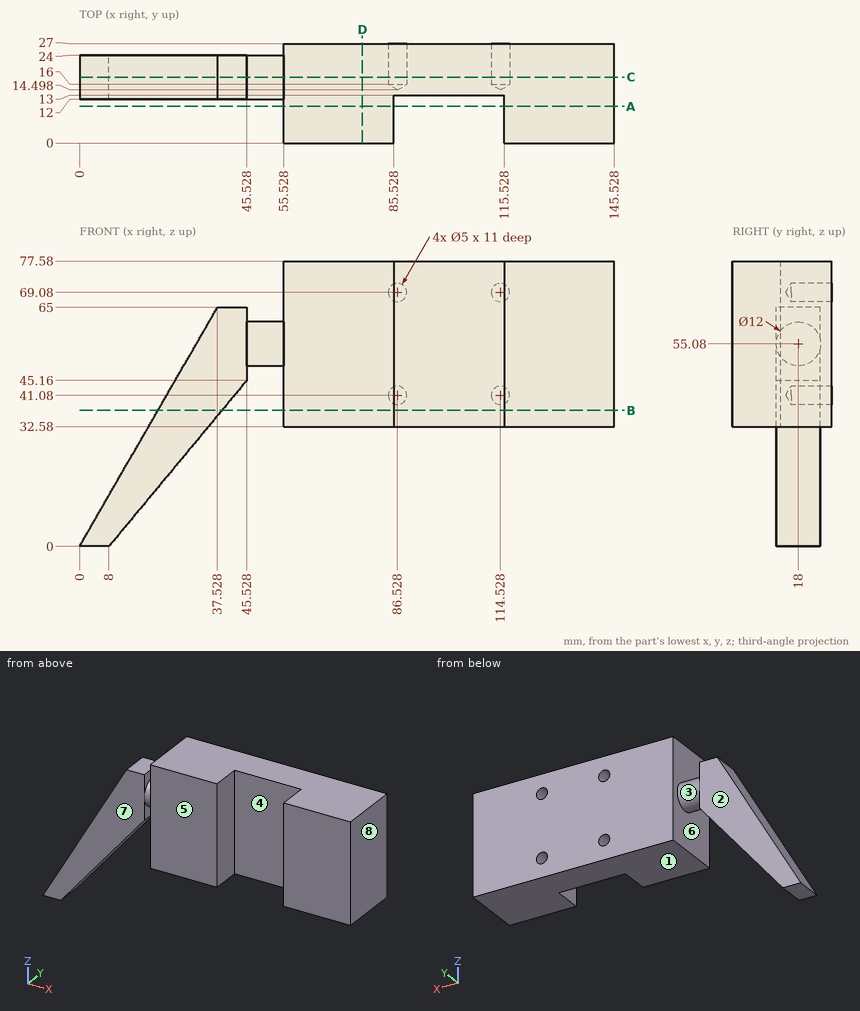
Design review of the part shown in the three views and the two pictorial views. Dimensions are in mm from the part's minimum x, y and z. A direction names the side the tool comes from. Round coordinates to 2 decimals unless told otherwise and drop trailing zeros. Loops run counter-clockwise (first coordinate to the right, second up) from the corner with the lowest first, then second, coordinate; pieces in that order, holes last.
Q1. Add section C-C on y = 18. Write out the cut boundary in (x, z), plus the area to 3 significant figures.
Result sheet:
outline: (0, 0) - (8, 0) - (45.53, 45.16) - (45.53, 49.08) - (55.53, 49.08) - (55.53, 32.58) - (145.53, 32.58) - (145.53, 77.58) - (55.53, 77.58) - (55.53, 61.08) - (45.53, 61.08) - (45.53, 65) - (37.53, 65) - close; hole circle Ø5 at (86.53, 41.08); hole circle Ø5 at (86.53, 69.08); hole circle Ø5 at (114.53, 41.08); hole circle Ø5 at (114.53, 69.08)
area: 4,980 mm2
Q2. Insertion check: pin 1 Ø14.5 at (y, z) = (5.5, 46.5) entering from -X; pin 2 Ø13.5 at (x, z) = (23, 19.5) entering from +Y; pin 3 Ø4 at (x, y) = (41, 20) entering from +Z. Each pin has a flat end and moves straight along its axis. Give the tip position at first contact, or say it passes through.
Result sheet:
pin 1: stops at x = 24.99
pin 2: stops at y = 24
pin 3: stops at z = 65
Q3. To check wall thickness, follow line 1 along X through (y, z) = (7.5, 67.5); line 2 along X through (y, z) = (19, 41) (1 decimal); line 3 along Z through (x, y) = (78, 11.25). State the ranges of each line that lie inside material, in increasing order.
Result sheet:
line 1: x = 55.53 to 85.53, 115.53 to 145.53
line 2: x = 23.7 to 42.1, 55.5 to 84, 89 to 112, 117 to 145.5
line 3: z = 32.58 to 77.58
Q4. Mouldability with a two-part tool opening along X and no side actions: class the marked faces 6, 7 and 8 as +X half, -X half, draft (parallel to the pull), parting line (faces both ways), or undercut.
Result sheet:
face 6: undercut
face 7: draft
face 8: +X half
Q5. Machinability: for the marked faces 1, 2, 3, 4 and 5, which of the approach directions +Z, -Z, +X, -X, +Y, -Y give a long, thin tool a straight path to every point of the face, cutting with its end or side? Answer none if there is none.
Result sheet:
face 1: -Z, +X, +Y, -Y
face 2: +Z, -Z, -X, +Y
face 3: none
face 4: +Z, -Z, -Y
face 5: +Z, -Z, +X, -X, -Y
Q6. Add section B-B on z = 37. Write out the cut boundary in (x, y), plus the area to 3 significant figures.
Result sheet:
outline: (21.36, 12) - (38.75, 12) - (38.75, 24) - (21.36, 24) - close; (55.53, 0) - (85.53, 0) - (85.53, 13) - (115.53, 13) - (115.53, 0) - (145.53, 0) - (145.53, 27) - (55.53, 27) - close
area: 2,250 mm2
Q7. Add section D-D on x = 77. Write out the cut boundary in (y, z), plus the area to 4 significant figures.
Result sheet:
outline: (0, 32.58) - (27, 32.58) - (27, 77.58) - (0, 77.58) - close
area: 1,215 mm2
Q8. Add section A-A on y = 10. Write out the cut boundary in (x, z), plus the area to 3 significant figures.
Result sheet:
outline: (55.53, 32.58) - (85.53, 32.58) - (85.53, 77.58) - (55.53, 77.58) - close; (115.53, 32.58) - (145.53, 32.58) - (145.53, 77.58) - (115.53, 77.58) - close
area: 2,700 mm2
